from build123d import *

# Parameters (mm, degrees)
SKETCH1_R           = 11.1125
SKETCH1_R_2         = 2.38125
BOSS_EXTRUDE1_DEPTH = 9.525
FILLET2_R           = 1.5875
CHAMFER2_SIZE       = 0.396875


with BuildPart() as part:
    # Sketch1 → Boss-Extrude1 (new body)
    with BuildSketch(Plane(origin=(0, 0, 0), x_dir=(1, 0, 0), z_dir=(0, 1, 0))):
        Circle(SKETCH1_R)
        Circle(SKETCH1_R_2, mode=Mode.SUBTRACT)
    extrude(amount=BOSS_EXTRUDE1_DEPTH)

    # Fillet2
    fillet2_edges = [part.edges().sort_by_distance(p)[0] for p in [
        (-11.1125, 0, 0),
        (-11.1125, 9.525, 0),
    ]]
    fillet(fillet2_edges, radius=FILLET2_R)

    # Chamfer2
    chamfer2_edges = [part.edges().sort_by_distance(p)[0] for p in [
        (-2.38125, 0, 0),
        (-2.38125, 9.525, 0),
    ]]
    chamfer(chamfer2_edges, length=CHAMFER2_SIZE)


solid = part.part
Can you work these out from the model? Positions are in its coordinate system, mm. Give positions to 0.01 mm unless a question says otherwise; leave off trailing zeros. Order: outer loops, then holes, each group sorted by start corner. A loop starts at its lowest first (then second) coordinate and runs counter-clockwise, first axis right, second up. Notation, with made-up numbers: M 35,20.25 L 90,20.25 A36 cw 90,56.25 Z; hole C -1,-40 d7. An arc over 180 degrees is marked long. One line per item, written item: value.
Item 1: Please list where these lines run through material, in increasing order: line 1 (X direction, y = 6.25, z = 0); line 2 (X direction, y = 1, z = -1).
Verdict:
line 1: -11.11 to -2.38, 2.38 to 11.11
line 2: -10.95 to -2.16, 2.16 to 10.95
Item 2: If we section it at B-B on z = 0: Write out the boundary of the cut face in (x, y) (1 decimal), and give its area (3 significant figures).
Verdict:
outline: M -11.1,1.6 A1.6 ccw -9.5,0 L -2.8,0 L -2.4,0.4 L -2.4,9.1 L -2.8,9.5 L -9.5,9.5 A1.6 ccw -11.1,7.9 Z; M 2.4,0.4 L 2.8,0 L 9.5,0 A1.6 ccw 11.1,1.6 L 11.1,7.9 A1.6 ccw 9.5,9.5 L 2.8,9.5 L 2.4,9.1 Z
area: 164 mm2
Item 3: If we section it at D-D on y = 8.5: Write out the boundary of the cut face in (x, z).
Verdict:
outline: C 0,0 d22.02; hole C 0,0 d4.76
Item 4: For pin 1 (1.5 mm diameter, centred on x = 8, z = 7.5, fed in from -Y); pin 2 (3 mm diameter, centred on y = 3, z = -6, fed in from -X); pin 3 (4 mm diameter, centred on y = 3.5, z = 4.5, fed in from +X), each with a flat end and sliding along its axis, tell me the tip position at first contact or that it passes through.
Verdict:
pin 1: y = 0.16
pin 2: x = -10.16
pin 3: x = 10.83
Item 5: If we section it at C-C on y = 7.25: Write out the boundary of the cut face in (x, z) (1 decimal), and give its area (3 significant figures).
Verdict:
outline: C 0,0 d22.2; hole C 0,0 d4.8
area: 370 mm2
Item 6: If we section it at A-A on x = 0: Write out the boundary of the cut face in (y, z) (1 decimal), and give its area (3 significant figures).
Verdict:
outline: M 0,-9.5 A1.6 ccw 1.6,-11.1 L 7.9,-11.1 A1.6 ccw 9.5,-9.5 L 9.5,-2.8 L 9.1,-2.4 L 0.4,-2.4 L 0,-2.8 Z; M 0,2.8 L 0.4,2.4 L 9.1,2.4 L 9.5,2.8 L 9.5,9.5 A1.6 ccw 7.9,11.1 L 1.6,11.1 A1.6 ccw 0,9.5 Z
area: 164 mm2
